from build123d import *

# Parameters (mm, degrees)
BOSS_EXTRUDE2_DEPTH = 2
BOSS_EXTRUDE3_DEPTH = 1
SKETCH4_W           = 9.2
SKETCH4_H           = 6.3
BOSS_EXTRUDE4_DEPTH = 1


with BuildPart() as part:
    # Sketch2 → Boss-Extrude2 (new body)
    with BuildSketch(Plane(origin=(0, 0, 0), x_dir=(1, 0, 0), z_dir=(0, 1, 0))):
        with BuildLine():
            Line((-2.5, 5.35), (-5.75, 5.35))
            Line((-5.75, 5.35), (-5.75, 2.8))
            Line((-5.75, 2.8), (-5.75, 0.25))
            Line((-5.75, 0.25), (-0.25, 0.25))
            Line((-0.25, 0.25), (-0.25, 2.8))
            ThreePointArc((-0.25, 2.8), (-0.977233386, 4.425970541), (-2.5, 5.35))
        make_face()
    extrude(amount=BOSS_EXTRUDE2_DEPTH)

    # Sketch3 → Boss-Extrude3 (add)
    with BuildSketch(Plane.XZ):
        with BuildLine():
            Line((-6.35, 0.35), (0.35, 0.35))
            Line((0.35, 0.35), (0.35, -2.8))
            ThreePointArc((0.35, -2.8), (-0.515014693, -4.881653373), (-2.5, -5.95))
            Line((-2.5, -5.95), (-6.35, -5.95))
            Line((-6.35, -5.95), (-6.35, 0.35))
        make_face()
    extrude(amount=BOSS_EXTRUDE3_DEPTH)

    # Sketch4 → Boss-Extrude4 (add)
    with BuildSketch(Plane.XZ.offset(1)):
        with Locations((-3, -2.8)):
            Rectangle(SKETCH4_W, SKETCH4_H)
    extrude(amount=BOSS_EXTRUDE4_DEPTH)


solid = part.part
CAD build for the part. Positions are in the model's coordinates, mm. A direction names the side the tool comes from. Give positions to 0.01 mm unless a question says otherwise; leave off trailing zeros. Write each loop counter-clockwise with the first axis right and the second up, starting at its lowest first coordinate (ties: lowest second). Pieces come first, ordered by that corner, then holes. Notation, with made-up numbers: (44.25, 53.25) - (86.25, 53.25) arc R17 cw to (86.25, 68.25) - close; hole circle Ø6 at (12, -12.5). An arc over 180 degrees is marked (long way). Put each result on its own line as item: value.
(1) Saw through at D-D (z = -1.5). List the corners of the cut face in (x, y), then the cut area to 3 significant figures.
Working result:
outline: (-7.6, -2) - (1.6, -2) - (1.6, -1) - (0.35, -1) - (0.35, 0) - (-0.25, 0) - (-0.25, 2) - (-5.75, 2) - (-5.75, 0) - (-6.35, 0) - (-6.35, -1) - (-7.6, -1) - close
area: 26.9 mm^2
(2) Saw through at C-C (x = -5.5). List the corners of the cut face in (y, z), then the cut area to 3 significant figures.
Working result:
outline: (-2, -5.95) - (0, -5.95) - (0, -5.35) - (2, -5.35) - (2, -0.25) - (0, -0.25) - (0, 0.35) - (-2, 0.35) - close
area: 22.8 mm^2
(3) Drop flat-ended pins along their axis: pin 1 Ø1.6 at (y, z) = (1, -1.5) entering from +X; pin 2 Ø1.4 at (x, z) = (-7, -2.5) entering from +Y; pin 3 Ø2 at (y, z) = (0.5, -2.5) entering from -X. Give the stop position or say it passes through.
Working result:
pin 1: x = -0.25
pin 2: y = 0
pin 3: x = -6.35
(4) Saw through at B-B (z = 0). List the corners of the cut face in (x, y), then the cut area to 3 significant figures.
Working result:
outline: (-7.6, -2) - (1.6, -2) - (1.6, -1) - (0.35, -1) - (0.35, 0) - (-6.35, 0) - (-6.35, -1) - (-7.6, -1) - close
area: 15.9 mm^2
(5) Wall check: L1, parallel to Y at x = -0.75, z = 0; L2, parallel to Z at x = -3.25, y = 1.6; L3, parallel to Y at x = 0.5, z = -5.5. Give the ranges that are in metal, low to high.
Working result:
L1: -2 to 0
L2: -5.35 to -0.25
L3: -2 to -1
(6) Tool access for faces 1 (the flat face through (-6.35, -0.5, -2.8)), 2 (the flat face through (0.35, -0.5, -1.2)), 3 (the cylindrical face through (-0.961, 0.986, -4.407)): list every direction of +Z, -Z, +X, -X, +Y, -Y with a clear straight run to the whole face (end or side of a thin tool).
Working result:
face 1: +Z, -Z, -X, +Y
face 2: +Z, -Z, +X, +Y
face 3: -Z, +X, +Y
(7) Saw through at A-A (y = 0.1). List the corners of the cut face in (x, z).
Working result:
outline: (-5.75, -5.35) - (-2.5, -5.35) arc R2.99 ccw to (-0.25, -2.8) - (-0.25, -0.25) - (-5.75, -0.25) - close
